```python
from build123d import *

# Parameters (mm, degrees)
F0_R     = 3.175
F1_DEPTH = 3.048


with BuildPart() as f1:
    # F0 (on Front) → F1 (new body)
    with BuildSketch(Plane.XZ):
        with BuildLine():
            Line((15.06596, -8.46577), (15.741248, -1.746608))
            ThreePointArc((15.741248, -1.746608), (0.511091, -16.085167), (-15.710986, -2.879252))
            Line((-15.710986, -2.879252), (-9.581655, -63.981123))
            ThreePointArc((-9.581655, -63.981123), (-0.19057, -54.196342), (9.464778, -63.72045))
            ThreePointArc((9.464778, -63.72045), (6.866195, -70.258827), (0.488322, -73.229642))
            Line((0.488322, -73.229642), (46.577481, -71.975364))
            ThreePointArc((46.577481, -71.975364), (38.36044, -63.761697), (46.494992, -55.466328))
            Line((46.494992, -55.466328), (18.991247, -54.712712))
            ThreePointArc((18.991247, -54.712712), (13.239164, -52.018093), (11.296671, -45.970435))
            Line((11.296671, -45.970435), (15.06596, -8.46577))
        make_face()
        with BuildLine():
            ThreePointArc((-15.710986, -2.879252), (0.511091, -16.085167), (15.741248, -1.746608))
            ThreePointArc((15.741248, -1.746608), (15.796385, -0.984415), (15.814778, -0.22045))
            ThreePointArc((15.814778, -0.22045), (15.783216, 0.780095), (15.688656, 1.776662))
            ThreePointArc((15.688656, 1.776662), (-0.063198, 15.654549), (-15.809848, 1.770757))
            ThreePointArc((-15.809848, 1.770757), (-15.931636, -0.557888), (-15.710986, -2.879252))
        make_face()
        with Locations((-0.060222, -0.22045)):
            Circle(F0_R, mode=Mode.SUBTRACT)
        with BuildLine():
            ThreePointArc((9.464778, -63.72045), (-0.19057, -54.196342), (-9.581655, -63.981123))
            ThreePointArc((-9.581655, -63.981123), (-6.713551, -70.536522), (-0.090768, -73.245402))
            Line((-0.090768, -73.245402), (0.488322, -73.229642))
            ThreePointArc((0.488322, -73.229642), (6.866195, -70.258827), (9.464778, -63.72045))
        make_face()
        with Locations((-0.060222, -63.72045)):
            Circle(F0_R, mode=Mode.SUBTRACT)
        with BuildLine():
            Line((-9.56921, 51.131614), (-15.809848, 1.770757))
            ThreePointArc((-15.809848, 1.770757), (-0.063198, 15.654549), (15.688656, 1.776662))
            Line((15.688656, 1.776662), (9.459404, 50.899448))
            ThreePointArc((9.459404, 50.899448), (9.463434, 50.739521), (9.464778, 50.57955))
            ThreePointArc((9.464778, 50.57955), (-0.336371, 41.058553), (-9.56921, 51.131614))
        make_face()
        with Locations((-6.428017, 36.30475)):
            Circle(F0_R, mode=Mode.SUBTRACT)
        with BuildLine():
            Line((0.488322, -73.229642), (-0.090768, -73.245402))
            ThreePointArc((-0.090768, -73.245402), (0.198897, -73.241925), (0.488322, -73.229642))
        make_face()
        with BuildLine():
            ThreePointArc((9.237933, 52.645931), (-0.824684, 60.073823), (-9.56921, 51.131614))
            ThreePointArc((-9.56921, 51.131614), (-0.336371, 41.058553), (9.464778, 50.57955))
            ThreePointArc((9.464778, 50.57955), (9.463434, 50.739521), (9.459404, 50.899448))
            Line((9.459404, 50.899448), (9.237933, 52.645931))
        make_face()
        with Locations((-0.060222, 50.57955)):
            Circle(F0_R, mode=Mode.SUBTRACT)
        with BuildLine():
            Line((9.237933, 52.645931), (9.459404, 50.899448))
            ThreePointArc((9.459404, 50.899448), (9.389105, 51.777817), (9.237933, 52.645931))
        make_face()
        with BuildLine():
            Line((47.187497, -55.485303), (46.494992, -55.466328))
            ThreePointArc((46.494992, -55.466328), (38.36044, -63.761697), (46.577481, -71.975364))
            ThreePointArc((46.577481, -71.975364), (52.439104, -69.570986), (54.870337, -63.72045))
            ThreePointArc((54.870337, -63.72045), (52.651404, -58.089205), (47.187497, -55.485303))
        make_face()
        with Locations((46.615337, -63.72045)):
            Circle(F0_R, mode=Mode.SUBTRACT)
        with BuildLine():
            ThreePointArc((47.187497, -55.485303), (46.841444, -55.468548), (46.494992, -55.466328))
            Line((46.494992, -55.466328), (47.187497, -55.485303))
        make_face()
    extrude(amount=F1_DEPTH)


solid = f1.part
```
Input: part model. Units: mm. Frame: model coordinates. A direction names the side the tool comes from. Round coordinates to 2 decimals unless told otherwise and drop trailing zeros. Write each loop counter-clockwise with the first axis right and the second up, starting at its lowest first coordinate (ties: lowest second). Pieces come first, ordered by that corner, then holes. Notation, with made-up numbers: (12.25, -23.5) - (65.25, -23.5) arc R24 cw to (65.25, 8.5) - close; hole circle Ø10 at (53, 60.5). An arc over 180 degrees is marked (long way). Write item = value, one per line.
(1) Section query D-D on x = 7. Output: boundary loops of the cut face in (y, z), then the cut area to 3 significant figures.
Geometry check:
outline = (-3.05, -73.05) - (0, -73.05) - (0, 56.97) - (-3.05, 56.97) - close
area = 396 mm^2
(2) Contact query for flat-ended pins moving along their axis: pin 1 Ø1 at (y, z) = (-1, -8.5) entering from -X; pin 2 Ø1.5 at (y, z) = (-2.5, 18.5) entering from -X; pin 3 Ø1 at (x, y) = (13.5, -1) entering from -Z. Output: stop coordinate, or through.
Geometry check:
pin_1 = -15.2
pin_2 = -13.79
pin_3 = -72.89
(3) Section query A-A on x = -7.5. Output: boundary loops of the cut face in (y, z).
Geometry check:
outline = (-3.05, -69.67) - (0, -69.67) - (0, 33.32) - (-3.05, 33.32) - close; (-3.05, 39.29) - (0, 39.29) - (0, 56.53) - (-3.05, 56.53) - close
(4) Section query B-B on y = -1.75. State how many separate pieces and enclosed holes the cut face has, then the cut area to 3 significant figures.
Geometry check:
separate_pieces = 1
enclosed_holes = 5
area = 3,830 mm^2
(5) Pull-direction query (X, two-part tool) for faces 3 (the flat face through (3, 0, -20)), 4 (the flat face through (12.62, -1.5, 25.99)), 5 (the cylindrical face through (-0.75, -1.5, 47.48)), 6 (the cylindrical face through (-15.932, -1.503, -0.525)); classes: +X half, -X half, draft (parallel to the pull), parting line (faces both ways), or undercut.
Geometry check:
face_3 = draft
face_4 = +X half
face_5 = undercut
face_6 = -X half
(6) Section query C-C on z = 28.5. Output: boundary loops of the cut face in (x, y).
Geometry check:
outline = (-12.43, -3.05) - (12.3, -3.05) - (12.3, 0) - (-12.43, 0) - close
(7) Access query for faces 1 (the cylindrical face through (13.3, -1.503, -52.086)), 2 (the cylindrical face through (-6.79, -1.5, -70.46)). Directions: +Z, -Z, +X, -X, +Y, -Y. A direction counts if a zero-diameter tool reaches every point of the face in a straight line with its end or side. Return the directions, or none.
Geometry check:
face_1 = +X, +Y, -Y
face_2 = -Z, -X, +Y, -Y
(8) Material intervals for probe 1 along X at (y, z) = (-2.7, -62.5); probe 2 along Z at (x, y) = (2.5, -2.65); probe 3 along Z at (x, y) = (1.5, -2.65), sorted ascending.
Geometry check:
probe_1 = -9.73 to -2.99, 2.87 to 43.68, 49.55 to 54.78
probe_2 = -73.17 to -65.6, -61.84 to -2.1, 1.66 to 48.7, 52.46 to 59.75
probe_3 = -73.2 to -66.49, -60.96 to -2.99, 2.54 to 47.81, 53.34 to 59.98
